from build123d import *

# Parameters (mm, degrees)
EXTRUDE_START            = 1
SKETCH_1_R               = 25
EXTRUDE_1_DEPTH          = 4
SKETCH_4_R               = 25
SKETCH_4_R_2             = 2
EXTRUDE_3_DEPTH          = 1
SKETCH_6_R               = 2.5
SKETCH_8_R               = 25
SKETCH_8_R_2             = 19
EXTRUDE_4_DEPTH          = 5
SKETCH_11_R              = 9
EXTRUDE_6_DEPTH          = 2
REVOLVE_1_ANGLE          = 15
PATTERN_CIRCULAR_1_COUNT = 5
SKETCH_13_R              = 2.5


with BuildPart() as part:
    # 草图1 → 凸台-拉伸1 (new body)
    with BuildSketch(Plane.XY.offset(EXTRUDE_START)):
        Circle(SKETCH_1_R)
        Polygon((3.464101615, 6), (-3.464101615, 6), (-6.92820323, 0), (-3.464101615, -6), (3.464101615, -6), (6.92820323, 0), align=None, mode=Mode.SUBTRACT)
    extrude(amount=EXTRUDE_1_DEPTH)

    # 草图4 → 凸台-拉伸3 (add)
    with BuildSketch(Plane.XY.offset(5)):
        Circle(SKETCH_4_R)
        Circle(SKETCH_4_R_2, mode=Mode.SUBTRACT)
    extrude(amount=EXTRUDE_3_DEPTH)

    # 切除-扫描1: sweep along a curve in space
    with BuildLine() as sweep_1_path:
        ThreePointArc((25, 0, 1), (17.67766953, 17.67766953, 1), (0, 25, 1))
        ThreePointArc((0, 25, 1), (-17.67766953, 17.67766953, 1), (-25, 0, 1))
        ThreePointArc((-25, 0, 1), (-17.67766953, -17.67766953, 1), (0, -25, 1))
        ThreePointArc((0, -25, 1), (17.67766953, -17.67766953, 1), (25, 0, 1))
    # 草图6 → 切除-扫描1 (sweep, cut)
    with BuildSketch(Plane(origin=(0, 0, 0), x_dir=(1, 0, 0), z_dir=(0, 1, 0))):
        with Locations((-25, -3.5)):
            Circle(SKETCH_6_R)
    sweep(path=sweep_1_path.line, mode=Mode.SUBTRACT)

    # 草图8 → 凸台-拉伸4 (add)
    with BuildSketch(Plane(origin=(0, 0, 1), x_dir=(-1, 0, 0), z_dir=(0, 0, -1))):
        Circle(SKETCH_8_R)
        Circle(SKETCH_8_R_2, mode=Mode.SUBTRACT)
    extrude(amount=EXTRUDE_4_DEPTH)

    # 草图11 → 凸台-拉伸6 (add)
    with BuildSketch(Plane(origin=(0, 0, 1), x_dir=(-1, 0, 0), z_dir=(0, 0, -1))):
        with Locations(Location((0, 0, 0), (0, 0, 180))):
            Circle(SKETCH_11_R)
        Polygon((-3.464101615, 6), (-6.92820323, 0), (-3.464101615, -6), (3.464101615, -6), (6.92820323, 0), (3.464101615, 6), align=None, mode=Mode.SUBTRACT)
    extrude(amount=EXTRUDE_6_DEPTH)

    # 草图12 → 旋转1 (revolve)
    with BuildSketch(Plane(origin=(0, 0, 0), x_dir=(1, 0, 0), z_dir=(0, 1, 0))):
        with BuildLine():
            Line((19, 4), (19, -1))
            Line((19, -1), (9, -1))
            Line((9, -1), (9, 1))
            Line((9, 1), (9.392071205, 1))
            ThreePointArc((9.392071205, 1), (12.772046971, 1.385768449), (15.978171002, 2.52323149))
            Line((15.978171002, 2.52323149), (19, 4))
        make_face()
    revolve_1 = revolve(axis=Axis((0, 0, -23.418623899), (0, 0, 1)), revolution_arc=REVOLVE_1_ANGLE)

    # 阵列(圆周)1: 旋转1 ×5 about axis
    pattern_circular_1_axis = Axis((0, 0, 0), (0, 0, 1))
    for i in range(1, PATTERN_CIRCULAR_1_COUNT):
        add(revolve_1.rotate(pattern_circular_1_axis, i * 360 / PATTERN_CIRCULAR_1_COUNT))

    # 切除-扫描2: sweep along a curve in space
    with BuildLine() as sweep_2_path:
        ThreePointArc((-25, 0, -4), (-17.67766953, 17.67766953, -4), (0, 25, -4))
        ThreePointArc((0, 25, -4), (17.67766953, 17.67766953, -4), (25, 0, -4))
        ThreePointArc((25, 0, -4), (17.67766953, -17.67766953, -4), (0, -25, -4))
        ThreePointArc((0, -25, -4), (-17.67766953, -17.67766953, -4), (-25, 0, -4))
    # 草图13 → 切除-扫描2 (sweep, cut)
    with BuildSketch(Plane(origin=(0, 0, 0), x_dir=(1, 0, 0), z_dir=(0, 1, 0))):
        with Locations((-25, 1.5)):
            Circle(SKETCH_13_R)
    sweep(path=sweep_2_path.line, mode=Mode.SUBTRACT)


solid = part.part
Model file for the job. Use its own axes, mm. A direction names the side the tool comes from. Give positions to 0.01 mm unless a question says otherwise; leave off trailing zeros. Order: outer loops, then holes, each group sorted by start corner. A loop starts at its lowest first (then second) coordinate and runs counter-clockwise, first axis right, second up. Notation, with made-up numbers: M -35.75,19.5 L 1.25,19.5 A20 ccw 1.25,39.5 Z; hole C 39.25,-15 d5. An arc over 180 degrees is marked long. Put each result on its own line as item: value. Start each with the question number.
(1) Pin check, flat tips, straight feed: pin 1 Ø6 at (x, y) = (0, 5.5) entering from -Z; pin 2 Ø3.5 at (x, y) = (1.5, 2.5) entering from -Z; pin 3 Ø4.5 at (x, y) = (13.5, 8.5) entering from -Z. Stop position of each tip, or through.
(2) Drill centre lines: L1, parallel to X at y = 15, z = 0.25; L2, parallel to Y at x = 12, z = 0; L3, parallel to Z at x = 22, y = 6. Where is each one in solid material? Low to high. Write a range as [from, to].
(3) Pull direction Y, two halves, no side cores. Call faces 3 (the face through (0, -5, 6)), 4 (the face through (-15, -2, 1)): released by +Y, released by -Y, zero draft, split by the parting line, or undercut.
(4) Tool access for faces 1 (the face through (-0.434, -1.952, 5.493)), 2 (the face through (7.94, -4.24, 0.01)): list every direction of +Z, -Z, +X, -X, +Y, -Y with a clear straight run to the whole face (end or side of a thin tool).
(5) Band-saw the part on A-A on z = 3. Give the cut face in (x, y).
Results below:
1. pin 1: stops at z = -1
1. pin 2: stops at z = 5
1. pin 3: stops at z = 1
2. L1: x = [-17.72, -11.66], [0.79, 4.87], [11.66, 17.72]
2. L2: y = [-19.62, -14.73], [0, 3.22], [14.73, 19.62]
2. L3: z = [-4, -2.69], [-0.31, 2.31], [4.69, 6]
3. face 3: zero draft
3. face 4: undercut
4. face 1: +Z, -Z
4. face 2: -Z
5. outline: C 0,0 d45.1; hole M -6.93,0 L -3.46,-6 L 3.46,-6 L 6.93,0 L 3.46,6 L -3.46,6 Z
